from build123d import *
from OCP.BRepFilletAPI import BRepFilletAPI_MakeChamfer

# Parameters (mm, degrees)
EXTRUDE_1_DEPTH     = 13
SKETCH_2_R          = 2.5
CUT_EXTRUDE_1_DEPTH = 43.582742984
EXTRUDE_2_DEPTH     = 25
EXTRUDE_3_DEPTH     = 13
SKETCH_4_R          = 2.2
CUT_EXTRUDE_3_DEPTH = 44.087005002
CHAMFER_3_SIZE      = 0.8
CHAMFER_3_SIZE2     = 0.291176187


with BuildPart() as part:
    # 草图1 → 凸台-拉伸1 (new body)
    with BuildSketch(Plane.XY):
        Polygon((3, 10), (9, 10), (9, 30.8), (27.5, 30.8), (27.5, 35.8), (-27.5, 35.8), (-27.5, 30.8), (-9, 30.8), (-9, 10), (-3, 10), (-3, 7.8), (-5, 7.8), (-5, 6.5), (-4.5, 6), (4.5, 6), (5, 6.5), (5, 7.8), (3, 7.8), align=None)
    extrude(amount=EXTRUDE_1_DEPTH)

    # 草图2 → 切除-拉伸1 (cut, through all)
    with BuildSketch(Plane(origin=(0, 35.8, 0), x_dir=(1, 0, 0), z_dir=(0, 1, 0))):
        with Locations(Location((21, -6.5, 0), (0, 0, 270))):
            Circle(SKETCH_2_R)
        with Locations((-21, -6.5)):
            Circle(SKETCH_2_R)
    extrude(amount=-CUT_EXTRUDE_1_DEPTH, mode=Mode.SUBTRACT)

    # 草图1<10> → 凸台-拉伸2 (add)
    with BuildSketch(Plane.XY):
        Polygon((3, 10), (9, 10), (9, 14), (-9, 14), (-9, 10), (-3, 10), align=None)
    extrude(amount=-EXTRUDE_2_DEPTH)

    # 草图1<11> → 凸台-拉伸3 (add)
    with BuildSketch(Plane.XY):
        Polygon((3, 7.8), (5, 7.8), (5, 6.5), (4.5, 6), (-4.5, 6), (-5, 6.5), (-5, 7.8), (-3, 7.8), (-3, 10), (3, 10), align=None)
    extrude(amount=-EXTRUDE_3_DEPTH)

    # 草图4 → 切除-拉伸3 (cut, through all)
    with BuildSketch(Plane(origin=(0, 14, 0), x_dir=(1, 0, 0), z_dir=(0, 1, 0))):
        with Locations(Location((0, 20, 0), (0, 0, 270))):
            Circle(SKETCH_4_R)
    extrude(amount=-CUT_EXTRUDE_3_DEPTH, mode=Mode.SUBTRACT)

    # 倒角3: one chamfer whose edges measure the first distance from different faces: ONE call of the kernel's chamfer builder (chamfer() names one face for all edges)
    chamfer_3_edges_1 = [part.edges().sort_by_distance(p)[0] for p in [
        (-3, 8.9, 13),
    ]]
    chamfer_3_side_1 = [part.faces().sort_by_distance(p)[0] for p in [
        (-3, 8.9, 0),
    ]]
    chamfer_3_edges_2 = [part.edges().sort_by_distance(p)[0] for p in [
        (3, 8.9, 13),
    ]]
    chamfer_3_side_2 = [part.faces().sort_by_distance(p)[0] for p in [
        (3, 8.9, 0),
    ]]
    chamfer_3_edges_3 = [part.edges().sort_by_distance(p)[0] for p in [
        (4, 7.8, 13),
    ]]
    chamfer_3_side_3 = [part.faces().sort_by_distance(p)[0] for p in [
        (4, 7.8, 0),
    ]]
    chamfer_3_edges_4 = [part.edges().sort_by_distance(p)[0] for p in [
        (5, 7.15, 13),
    ]]
    chamfer_3_side_4 = [part.faces().sort_by_distance(p)[0] for p in [
        (5, 7.15, 0),
    ]]
    chamfer_3_edges_5 = [part.edges().sort_by_distance(p)[0] for p in [
        (4.75, 6.25, 13),
    ]]
    chamfer_3_side_5 = [part.faces().sort_by_distance(p)[0] for p in [
        (4.75, 6.25, 0),
    ]]
    chamfer_3_edges_6 = [part.edges().sort_by_distance(p)[0] for p in [
        (0, 6, 13),
    ]]
    chamfer_3_side_6 = [part.faces().sort_by_distance(p)[0] for p in [
        (0, 6, 0),
    ]]
    chamfer_3_edges_7 = [part.edges().sort_by_distance(p)[0] for p in [
        (-4, 7.8, 13),
    ]]
    chamfer_3_side_7 = [part.faces().sort_by_distance(p)[0] for p in [
        (-4, 7.8, 0),
    ]]
    chamfer_3_edges_8 = [part.edges().sort_by_distance(p)[0] for p in [
        (-5, 7.15, 13),
    ]]
    chamfer_3_side_8 = [part.faces().sort_by_distance(p)[0] for p in [
        (-5, 7.15, 0),
    ]]
    chamfer_3_edges_9 = [part.edges().sort_by_distance(p)[0] for p in [
        (-4.75, 6.25, 13),
    ]]
    chamfer_3_side_9 = [part.faces().sort_by_distance(p)[0] for p in [
        (-4.75, 6.25, 0),
    ]]
    chamfer_3 = BRepFilletAPI_MakeChamfer(part.part.solid().wrapped)
    for e in chamfer_3_edges_1:
        chamfer_3.Add(CHAMFER_3_SIZE, CHAMFER_3_SIZE2, e.wrapped, chamfer_3_side_1[0].wrapped)  # the first distance lies on this face
    for e in chamfer_3_edges_2:
        chamfer_3.Add(CHAMFER_3_SIZE, CHAMFER_3_SIZE2, e.wrapped, chamfer_3_side_2[0].wrapped)  # the first distance lies on this face
    for e in chamfer_3_edges_3:
        chamfer_3.Add(CHAMFER_3_SIZE, CHAMFER_3_SIZE2, e.wrapped, chamfer_3_side_3[0].wrapped)  # the first distance lies on this face
    for e in chamfer_3_edges_4:
        chamfer_3.Add(CHAMFER_3_SIZE, CHAMFER_3_SIZE2, e.wrapped, chamfer_3_side_4[0].wrapped)  # the first distance lies on this face
    for e in chamfer_3_edges_5:
        chamfer_3.Add(CHAMFER_3_SIZE, CHAMFER_3_SIZE2, e.wrapped, chamfer_3_side_5[0].wrapped)  # the first distance lies on this face
    for e in chamfer_3_edges_6:
        chamfer_3.Add(CHAMFER_3_SIZE, CHAMFER_3_SIZE2, e.wrapped, chamfer_3_side_6[0].wrapped)  # the first distance lies on this face
    for e in chamfer_3_edges_7:
        chamfer_3.Add(CHAMFER_3_SIZE, CHAMFER_3_SIZE2, e.wrapped, chamfer_3_side_7[0].wrapped)  # the first distance lies on this face
    for e in chamfer_3_edges_8:
        chamfer_3.Add(CHAMFER_3_SIZE, CHAMFER_3_SIZE2, e.wrapped, chamfer_3_side_8[0].wrapped)  # the first distance lies on this face
    for e in chamfer_3_edges_9:
        chamfer_3.Add(CHAMFER_3_SIZE, CHAMFER_3_SIZE2, e.wrapped, chamfer_3_side_9[0].wrapped)  # the first distance lies on this face
    add(Compound.cast(chamfer_3.Shape()), mode=Mode.REPLACE)


solid = part.part
Geometry check sheet. Reference: the model listing, model coordinates, mm. A direction names the side the tool comes from. Give positions to 0.01 mm unless a question says otherwise; leave off trailing zeros. Order: outer loops, then holes, each group sorted by start corner. A loop starts at its lowest first (then second) coordinate and runs counter-clockwise, first axis right, second up.
1. Sectioned sample at C-C (y = 12.25). Record the boundary of the cut face in (x, z).
Completed:
outline: (-9, -25) - (9, -25) - (9, 13) - (-9, 13) - close; hole circle Ø4.4 at (0, -20)
2. Sectioned sample at A-A (z = 6.5). Record the boundary of the cut face in (x, y), then the cut area to 3 significant figures.
Completed:
outline: (-27.5, 30.8) - (-23.5, 30.8) - (-23.5, 35.8) - (-27.5, 35.8) - close; (-18.5, 30.8) - (-9, 30.8) - (-9, 10) - (-3, 10) - (-3, 7.8) - (-5, 7.8) - (-5, 6.5) - (-4.5, 6) - (4.5, 6) - (5, 6.5) - (5, 7.8) - (3, 7.8) - (3, 10) - (9, 10) - (9, 30.8) - (18.5, 30.8) - (18.5, 35.8) - (-18.5, 35.8) - close; (23.5, 30.8) - (27.5, 30.8) - (27.5, 35.8) - (23.5, 35.8) - close
area: 630 mm2
3. Draft check along Z on faces 4 (the face through (-23.5, 33.3, 6.4)), 5 (the face through (0, 35.8, 6)), 6 (the face through (0, 8, -13)), 7 (the face through (-0.843, 12.028, -17.968)). Enter one of: pulls with the +Z half, pulls with the -Z half, needs draft (parallel to the pull), parting line crosses it, or undercut.
Completed:
face 4: undercut
face 5: needs draft
face 6: pulls with the -Z half
face 7: undercut
4. Depth check by flat-ended pin: pin 1 (2.5 mm diameter, centred on y = 9.5, z = -4.5, fed in from -X); pin 2 (20 mm diameter, centred on x = 2, z = -16, fed in from +Y); pin 3 (10 mm diameter, centred on x = 14.5, z = -16.5, fed in from -Y); pin 4 (1.5 mm diameter, centred on x = -8, y = 25.5, fed in from -Z). Enter the tip coordinate at first touch or a pass-through.
Completed:
pin 1: stops at x = -9
pin 2: stops at y = 14
pin 3: passes through
pin 4: stops at z = 0
5. Sectioned sample at D-D (z = -20). Record the boundary of the cut face in (x, y).
Completed:
outline: (-9, 10) - (-2.2, 10) - (-2.2, 14) - (-9, 14) - close; (2.2, 10) - (9, 10) - (9, 14) - (2.2, 14) - close
6. Access from +Z, -Z, +X, -X, +Y, -Y to the whole of each face (thin tool, end or side, straight path). Record for faces 1 (the face through (5, 7, 0)), 2 (the face through (-4, 7.8, 0)), 3 (the face through (-18, 30.8, 6)).
Completed:
face 1: +Z, -Z, +X, -Y
face 2: +Z, -Z, -X
face 3: +Z, -Z, -X, -Y
7. Sectioned sample at B-B (x = 0). Record the boundary of the cut face in (y, z).
Completed:
outline: (6, -13) - (10, -13) - (10, -17.8) - (14, -17.8) - (14, 0) - (35.8, 0) - (35.8, 13) - (6.29, 13) - (6, 12.2) - close; (10, -25) - (14, -25) - (14, -22.2) - (10, -22.2) - close
8. Scan lines: line 1 (X direction, y = 33.1, z = 6.5); line 2 (X direction, y = 11.4, z = -20); line 3 (Y direction, x = -15.5, z = 0.5). Record each from-to range of solid material in increasing order.
Completed:
line 1: x = -27.5 to -23.5, -18.5 to 18.5, 23.5 to 27.5
line 2: x = -9 to -2.2, 2.2 to 9
line 3: y = 30.8 to 35.8
